Model file for the job. Use its own axes, mm. Face numbers are marked on the shaded views. A direction names the side the tool comes from. Round coordinates to 2 decimals unless told otherwise and drop trailing zeros. Write each loop counter-clockwise with the first axis right and the second up, starting at its lowest first coordinate (ties: lowest second). Pieces come first, ordered by that corner, then holes.
```python
from build123d import *

# Parameters (mm, degrees)
F0_R     = 5
F1_ANGLE = 45
F2_R     = 17.5
F2_R_2   = 5
F3_DEPTH = 1
F5_ANGLE = 135
F7_ANGLE = 45
F8_R     = 5
F9_R     = 5


with BuildPart() as f1:
    # F0 (on Top) → F1 (revolve)
    with BuildSketch(Plane.XY):
        with Locations((17.2625295818, 39.9485491216)):
            Circle(F0_R)
    revolve(axis=Axis((11.3439466804, 38.7977138162, 0), (0, -1, 0)), revolution_arc=F1_ANGLE)

    # F2 (on face) → F3 (join)
    with BuildSketch(Plane(origin=(0, 0, 0), x_dir=(1, 0, 0), z_dir=(0, 0, -1))):
        with Locations((17.2625295818, -39.9485491216)):
            Circle(F2_R)
        with Locations((17.2625295818, -39.9485491216)):
            Circle(F2_R_2, mode=Mode.SUBTRACT)
        with Locations((17.2625295818, -39.9485491216)):
            Circle(F2_R_2)
    extrude(amount=F3_DEPTH)

    # F4 (on face) → F5 (revolve)
    with BuildSketch(Plane(origin=(0, 0, -1), x_dir=(1, 0, 0), z_dir=(0, 0, -1))):
        Polygon((12.9011229654, -29.9485491216), (2.9011229654, -29.9485491216), (2.9011229654, -49.9485491216), (12.9011229654, -49.9485491216), (12.9011229654, -44.1824280606), (21.6239361981, -44.1824280606), (21.6239361981, -49.9485491216), (31.6239361981, -49.9485491216), (31.6239361981, -29.9485491216), (21.6239361981, -29.9485491216), (21.6239361981, -36.1191299331), (12.9011229654, -36.1218505295), align=None)
    revolve(axis=Axis((-26.9732894376, 40.484293364, -1), (0, 1, 0)), revolution_arc=F5_ANGLE)

    # F6 (on face) → F7 (revolve)
    with BuildSketch(Plane(origin=(-12.9866447188, 0, 12.9866447188), x_dir=(0, -1, 0), z_dir=(-0.7071067812, 0, 0.7071067812))):
        Polygon((-36.1218505295, -59.6545150564), (-29.9485491216, -59.6545150564), (-29.9485491216, -49.6545150564), (-49.9485491216, -49.6545150564), (-49.9485491216, -59.6545150564), (-44.1824280606, -59.6545150564), (-44.1824280606, -68.3773282891), (-49.9485491216, -68.3773282891), (-49.9485491216, -78.3773282891), (-29.9485491216, -78.3773282891), (-29.9485491216, -68.3773282891), (-36.1191299331, -68.3773282891), align=None)
    revolve(axis=Axis((-83.5220088064, 42.3686988652, -57.5487193688), (0, -1, 0)), revolution_arc=F7_ANGLE)

    # F8
    f8_edges = [f1.edges().sort_by_distance(p)[0] for p in [
        (-83.522009, 39.948549, -36.173979),
    ]]
    fillet(f8_edges, radius=F8_R)

    # F9
    f9_edges = [f1.edges().sort_by_distance(p)[0] for p in [
        (-83.522009, 39.948549, -7.451166),
    ]]
    fillet(f9_edges, radius=F9_R)


solid = f1.part
```
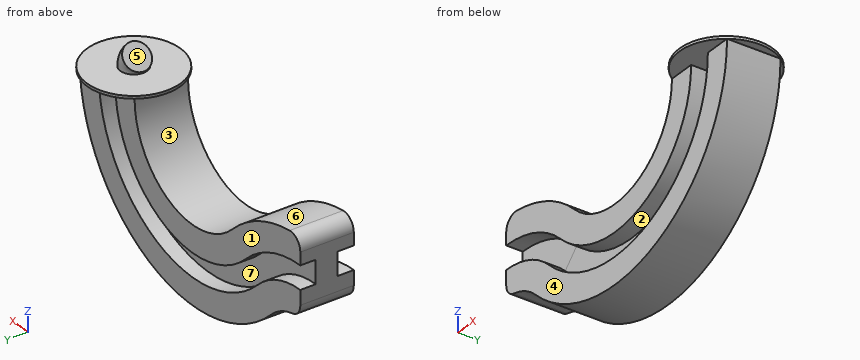
1) Which spindle directions (+Z, -Z, +X, -X, +Y, -Y) get a long thin tool onto all of the face, cutting with end or side? Do the marked faces 1, 2 and 3. Say none if no direction does.
2) Cut at B-B on x = 26.5. List the corners of the cut face in (y, z), and give its area (3 significant figures).
3) Wall check: probe 1 along Y at (x, z) = (-21.5, -38.5); probe 2 along Z at (x, y) = (-70.5, 31); probe 3 along X at (y, z) = (31.5, -35). Give the ranges that are in metal, low to high.
4) Cut at D-D on y = 53. List the corners of the cut face in (x, z), and give its area (3 significant figures).
5) Pull direction X, two halves, no side cores. Call the marked faces 4, 5, 6 and 7: released by +X, released by -X, zero draft, split by the parting line, or undercut.
6) Cut at A-A on y = 42.5. List the corners of the cut face in (x, z), and give its area (3 significant figures).
7) Cut at C-C on y = 48. List the corners of the cut face in (x, z), and give its area (3 significant figures).
8) Flat gauge pins, fed straight in: pin 1 Ø10.5 at (x, y) = (21.5, 33.5) entering from +Z; pin 2 Ø14.5 at (x, y) = (16.5, 50.5) entering from -Z; pin 3 Ø6 at (x, z) = (2, -48) entering from -Y; pin 4 Ø24.5 at (x, z) = (-22.5, -13.5) entering from +Y. Where does each tip first touch, or does it go through?
Result sheet:
1. face 1: -Z, +X, -X, +Y
1. face 2: -Y
1. face 3: +Y, -Y
2. outline: (25.09, -1) - (29.95, -1) - (29.95, -24.96) - (49.95, -24.96) - (49.95, -1) - (54.81, -1) - (54.81, 0) - (25.09, 0) - close
2. area: 509 mm2
3. probe 1: y = 29.95 to 49.95
3. probe 2: z = -40.6 to -29, -19.62 to -9.17
3. probe 3: x = -82.24 to -61.71, -47.81 to -6.14, 7.75 to 20.75
4. outline: (5.6, -1) - (28.92, -1) - (28.92, 0) - (5.6, 0) - close
4. area: 23.3 mm2
5. face 4: zero draft
5. face 5: released by -X
5. face 6: undercut
5. face 7: undercut
6. outline: (-83.52, -31.65) arc R5 ccw to (-79.47, -36.56) arc R21.37 cw to (-68.41, -42.43) arc R58.6 ccw to (31.62, -1) - (34.58, -1) - (34.58, 0) - (21.56, 0) arc R10.22 ccw to (18.57, 7.23) - (12.49, 1.14) arc R1.62 cw to (12.96, 0) - (-0.05, 0) - (-0.05, -1) - (2.9, -1) arc R29.87 cw to (-48.1, -22.12) arc R50.1 ccw to (-77.97, -7.76) arc R5 ccw to (-83.52, -12.73) - close
6. area: 3,860 mm2
7. outline: (-83.52, -31.65) arc R5 ccw to (-79.47, -36.56) arc R21.37 cw to (-68.41, -42.43) arc R58.6 ccw to (31.62, -1) - (32.8, -1) - (32.8, 0) - (1.72, 0) - (1.72, -1) - (2.9, -1) arc R29.87 cw to (-48.1, -22.12) arc R50.1 ccw to (-77.97, -7.76) arc R5 ccw to (-83.52, -12.73) - (-83.52, -17.45) arc R40.1 cw to (-55.17, -29.2) arc R39.87 ccw to (12.9, -1) - (21.62, -1) arc R48.6 cw to (-61.34, -35.36) arc R31.37 ccw to (-83.52, -26.17) - close
7. area: 2,670 mm2
8. pin 1: stops at z = 7.44
8. pin 2: stops at z = -47.04
8. pin 3: stops at y = 29.95
8. pin 4: passes through
